Can you work these out from the drawing? Everything is in mm from the part's minimum corner. Coordinates: 2 decimals unless noted, no trailing zeros. Loops run counter-clockwise (first coordinate to the right, second up) from the corner with the lowest first, then second, coordinate; pieces in that order, holes last. Notation, with made-up numbers: (-10.75, 58.25) -> (22.25, 58.25) arc R17 ccw to (22.25, 65.25) -> close; hole circle Ø10 at (10, 69.25). An arc over 180 degrees is marked (long way). Use one line per item in the form item = value. Start each with the question number.
(1) Imagine slicing it at B-B (y = 90.64). List the corners of the cut face in (x, z) for me.
(2) Imagine slicing it at C-C (x = 52.5). List the corners of the cut face in (y, z) for me, plus the area to 3 significant figures.
(3) Thinking about a two-plate mould opening in Z: for the marked faces 1 and 2, which applies, released by +Z, released by -Z, zero draft, split by the parting line, or undercut?
(4) I'm going to push a flat-ended pin straight in: pin 1 (2.5 mm diameter, centred on x = 22.5, y = 50, fed in from +Z). Where does the tip first touch, or does it pass through?
(5) Imagine slicing it at A-A (x = 75.8). List the corners of the cut face in (y, z) for me.
(6) I need wall thicknesses on line 1 (X direction, y = 90.64, z = 0.7); line 2 (Y direction, x = 75.8, z = 2.05); line 3 (Y direction, x = 52.5, z = 0.8). Which ranges of each line are inside material? Lowest first, please. Write a range as [from, to].
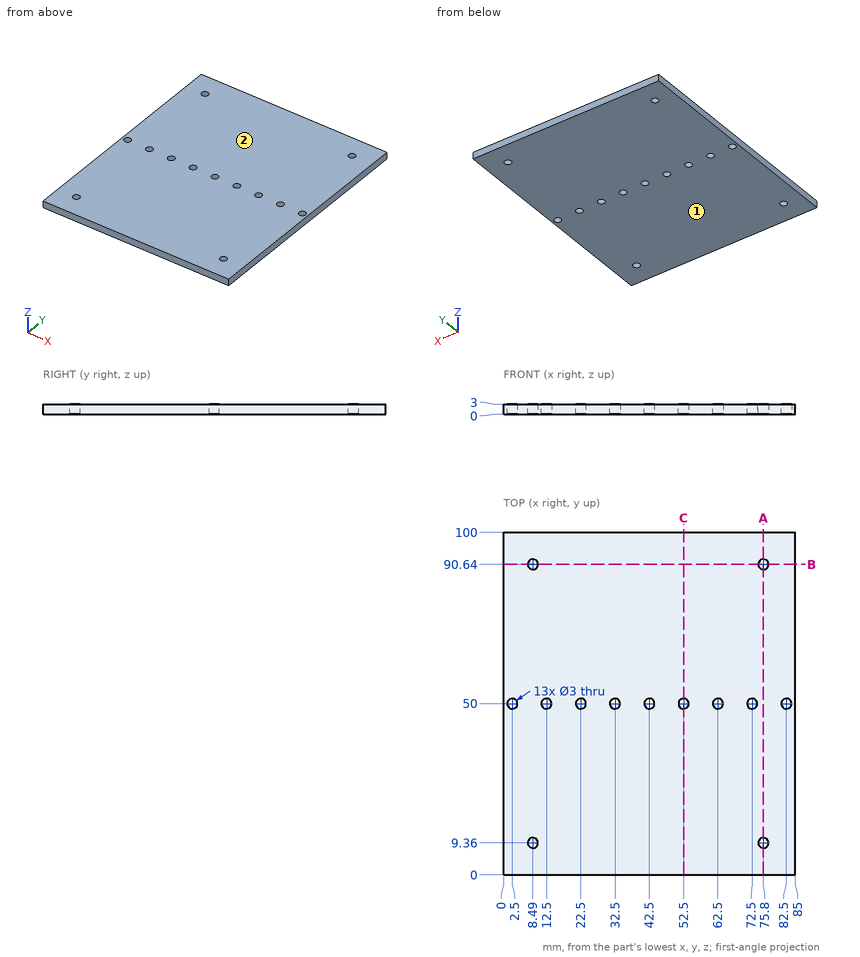
Worked out:
q1.outline = (0, 0) -> (6.99, 0) -> (6.99, 3) -> (0, 3) -> close; (9.99, 0) -> (74.3, 0) -> (74.3, 3) -> (9.99, 3) -> close; (77.3, 0) -> (85, 0) -> (85, 3) -> (77.3, 3) -> close
q2.outline = (0, 0) -> (48.5, 0) -> (48.5, 3) -> (0, 3) -> close; (51.5, 0) -> (100, 0) -> (100, 3) -> (51.5, 3) -> close
q2.area = 291 mm2
q3.face_1 = released by -Z
q3.face_2 = released by +Z
q4.pin_1 = through
q5.outline = (0, 0) -> (7.86, 0) -> (7.86, 3) -> (0, 3) -> close; (10.86, 0) -> (89.14, 0) -> (89.14, 3) -> (10.86, 3) -> close; (92.14, 0) -> (100, 0) -> (100, 3) -> (92.14, 3) -> close
q6.line_1 = [0, 6.99], [9.99, 74.3], [77.3, 85]
q6.line_2 = [0, 7.86], [10.86, 89.14], [92.14, 100]
q6.line_3 = [0, 48.5], [51.5, 100]
